Part model, mm, in its own coordinate system. A direction names the side the tool comes from. Coordinates: 2 decimals unless noted, no trailing zeros. Loops run counter-clockwise (first coordinate to the right, second up) from the corner with the lowest first, then second, coordinate; pieces in that order, holes last. Notation, with made-up numbers: M -34,-18.75 L 1,-18.75 A29 cw 1,4.25 Z; hole C 84.25,61 d5. An arc over 180 degrees is marked long. Use CSV: the item, a comma, the result in double quotes. Start each with the question number.
from build123d import *

# Parameters (mm, degrees)
SKETCH1_W                      = 60
SKETCH1_H                      = 42
BOSS_EXTRUDE1_DEPTH            = 12
CUT_EXTRUDE1_REACH             = 14
SKETCH2_R                      = 4
CUT_EXTRUDE1_DIRECTION_2_DEPTH = 1
SKETCH3_R                      = 8
SKETCH3_R_2                    = 4
CUT_EXTRUDE2_DEPTH             = 1
CUT_EXTRUDE2_DEPTH_BACK        = 10
CHAMFER1_SIZE                  = 13
CUT_EXTRUDE4_REACH             = 14
SKETCH5_W                      = 7
SKETCH5_H                      = 4
CUT_EXTRUDE4_DIRECTION_2_DEPTH = 1
SKETCH4_R                      = 2.25
CUT_EXTRUDE3_DEPTH             = 7.5


with BuildPart() as part:
    # Sketch1 → Boss-Extrude1 (new body)
    with BuildSketch(Plane(origin=(0, 0, 0), x_dir=(1, 0, 0), z_dir=(0, 1, 0))):
        Rectangle(SKETCH1_W, SKETCH1_H)
    extrude(amount=BOSS_EXTRUDE1_DEPTH)

    # Sketch2 → Cut-Extrude1 (cut, up to next)
    with BuildSketch(Plane(origin=(0, 12, 0), x_dir=(1, 0, 0), z_dir=(0, 1, 0)), mode=Mode.PRIVATE) as cut_extrude1_sk1:
        Circle(SKETCH2_R)
    cut_extrude1_tool1 = extrude(cut_extrude1_sk1.sketch, amount=-CUT_EXTRUDE1_REACH, mode=Mode.PRIVATE) & part.part
    add(cut_extrude1_tool1.solids().sort_by_distance((0, 12, 0))[0], mode=Mode.SUBTRACT)

    # Sketch2 → Cut-Extrude1 direction 2 (cut)
    with BuildSketch(Plane(origin=(0, 12, 0), x_dir=(1, 0, 0), z_dir=(0, 1, 0))):
        Circle(SKETCH2_R)
    extrude(amount=CUT_EXTRUDE1_DIRECTION_2_DEPTH, mode=Mode.SUBTRACT)

    # Sketch3 → Cut-Extrude2 (cut, two sides)
    with BuildSketch(Plane(origin=(0, 12, 0), x_dir=(1, 0, 0), z_dir=(0, 1, 0))) as cut_extrude2_sk:
        Circle(SKETCH3_R)
        with Locations((20.75, 0)):
            Circle(SKETCH3_R_2)
        with Locations((-20.75, 0)):
            Circle(SKETCH3_R_2)
    extrude(amount=CUT_EXTRUDE2_DEPTH, mode=Mode.SUBTRACT)
    extrude(cut_extrude2_sk.sketch, amount=-CUT_EXTRUDE2_DEPTH_BACK, mode=Mode.SUBTRACT)

    # Chamfer1
    chamfer1_edges = [part.edges().sort_by_distance(p)[0] for p in [
        (30, 6, 21),
        (-30, 6, 21),
    ]]
    chamfer(chamfer1_edges, length=CHAMFER1_SIZE)

    # Sketch5 → Cut-Extrude4 (cut, up to next)
    with BuildSketch(Plane(origin=(0, 12, 0), x_dir=(1, 0, 0), z_dir=(0, 1, 0)), mode=Mode.PRIVATE) as cut_extrude4_sk1:
        with Locations((24, 15)):
            Rectangle(SKETCH5_W, SKETCH5_H)
    cut_extrude4_tool1 = extrude(cut_extrude4_sk1.sketch, amount=-CUT_EXTRUDE4_REACH, mode=Mode.PRIVATE) & part.part
    add(cut_extrude4_tool1.solids().sort_by_distance((24, 12, -15))[0], mode=Mode.SUBTRACT)
    # Sketch5 → Cut-Extrude4 (cut, up to next)
    with BuildSketch(Plane(origin=(0, 12, 0), x_dir=(1, 0, 0), z_dir=(0, 1, 0)), mode=Mode.PRIVATE) as cut_extrude4_sk2:
        with Locations((6, 15)):
            Rectangle(SKETCH5_W, SKETCH5_H)
    cut_extrude4_tool2 = extrude(cut_extrude4_sk2.sketch, amount=-CUT_EXTRUDE4_REACH, mode=Mode.PRIVATE) & part.part
    add(cut_extrude4_tool2.solids().sort_by_distance((6, 12, -15))[0], mode=Mode.SUBTRACT)
    # Sketch5 → Cut-Extrude4 (cut, up to next)
    with BuildSketch(Plane(origin=(0, 12, 0), x_dir=(1, 0, 0), z_dir=(0, 1, 0)), mode=Mode.PRIVATE) as cut_extrude4_sk3:
        with Locations((-6, 15)):
            Rectangle(SKETCH5_W, SKETCH5_H)
    cut_extrude4_tool3 = extrude(cut_extrude4_sk3.sketch, amount=-CUT_EXTRUDE4_REACH, mode=Mode.PRIVATE) & part.part
    add(cut_extrude4_tool3.solids().sort_by_distance((-6, 12, -15))[0], mode=Mode.SUBTRACT)
    # Sketch5 → Cut-Extrude4 (cut, up to next)
    with BuildSketch(Plane(origin=(0, 12, 0), x_dir=(1, 0, 0), z_dir=(0, 1, 0)), mode=Mode.PRIVATE) as cut_extrude4_sk4:
        with Locations((-24, 15)):
            Rectangle(SKETCH5_W, SKETCH5_H)
    cut_extrude4_tool4 = extrude(cut_extrude4_sk4.sketch, amount=-CUT_EXTRUDE4_REACH, mode=Mode.PRIVATE) & part.part
    add(cut_extrude4_tool4.solids().sort_by_distance((-24, 12, -15))[0], mode=Mode.SUBTRACT)

    # Sketch5 → Cut-Extrude4 direction 2 (cut)
    with BuildSketch(Plane(origin=(0, 12, 0), x_dir=(1, 0, 0), z_dir=(0, 1, 0))):
        with Locations((24, 15)):
            Rectangle(SKETCH5_W, SKETCH5_H)
        with Locations((6, 15)):
            Rectangle(SKETCH5_W, SKETCH5_H)
        with Locations((-6, 15)):
            Rectangle(SKETCH5_W, SKETCH5_H)
        with Locations((-24, 15)):
            Rectangle(SKETCH5_W, SKETCH5_H)
    extrude(amount=CUT_EXTRUDE4_DIRECTION_2_DEPTH, mode=Mode.SUBTRACT)

    # Sketch4 → Cut-Extrude3 (cut)
    with BuildSketch(Plane(origin=(0, 0, -21), x_dir=(-1, 0, 0), z_dir=(0, 0, -1))):
        with Locations((-24, 6)):
            Circle(SKETCH4_R)
        with Locations((-6, 6)):
            Circle(SKETCH4_R)
        with Locations((6, 6)):
            Circle(SKETCH4_R)
        with Locations((24, 6)):
            Circle(SKETCH4_R)
    extrude(amount=-CUT_EXTRUDE3_DEPTH, mode=Mode.SUBTRACT)


solid = part.part
1. Wall check: probe 1 along X at (y, z) = (8.75, 0); probe 2 along Z at (x, y) = (8.5, 10.25); probe 3 along Y at (x, z) = (24, -18). Give the ranges that are in metal, low to high.
2. Two-plate mould, pull along Y, no slides. Class faces 1 (the face through (0, 6, 21)), 2 (the face through (-26.146, 6.676, -19.028)), 3 (the face through (-4, 2, 2)): pulls with the +Y half, pulls with the -Y half, needs draft (parallel to the pull), parting line crosses it, or undercut.
3. Tool access for faces 4 (the face through (0, 0, -5)), 5 (the face through (6, 6, -13)), 6 (the face through (-7, 12, -5)), 7 (the face through (-8.146, 6.676, -19.028)), 8 (the face through (-21, 2, 0)): list every direction of +Z, -Z, +X, -X, +Y, -Y with a clear straight run to the whole face (end or side of a thin tool).
4. Slice it at A-A, the plane x = 0. List the corners of the cut face in (y, z), and give its area (3 significant figures).
5. Pin check, flat tips, straight feed: pin 1 (7 mm diameter, centred on x = -24, y = 6, fed in from +Z); pin 2 (8 mm diameter, centred on x = 2, z = -2, fed in from +Y); pin 3 (3.5 mm diameter, centred on x = -24, y = 7.5, fed in from +Z). Stop position of each tip, or through.
6. Slice it at C-C, the plane z = 0. List the corners of the cut face in (x, y).
7. Slice it at B-B, the plane z = -15.5. List the corners of the cut face in (x, y), and give its area (3 significant figures).
8. Slice it at D-D, the plane y = 10.5. List the corners of the cut face in (x, z), and give its area (3 significant figures).
Found:
1,probe 1,"-30 to -24.75, -16.75 to -8, 8 to 16.75, 24.75 to 30"
1,probe 2,"-21 to -17, -13 to 21"
1,probe 3,"0 to 3.75, 8.25 to 12"
2,face 1,"needs draft"
2,face 2,"undercut"
2,face 3,"pulls with the +Y half"
3,face 4,"+Z, -Z, +X, -X, -Y"
3,face 5,"+Y, -Y"
3,face 6,"+Z, -Z, +X, -X, +Y"
3,face 7,"-Z"
3,face 8,"+Y"
4,outline,"M 0,-21 L 12,-21 L 12,-8 L 2,-8 L 2,-4 L 0,-4 Z; M 0,4 L 2,4 L 2,8 L 12,8 L 12,21 L 0,21 Z"
4,area,"328 mm^2"
5,pin 1,"z = 17.5"
5,pin 2,"y = 2"
5,pin 3,"z = 15.75"
6,outline,"M -30,0 L -4,0 L -4,2 L -8,2 L -8,12 L -16.75,12 L -16.75,2 L -24.75,2 L -24.75,12 L -30,12 Z; M 4,0 L 30,0 L 30,12 L 24.75,12 L 24.75,2 L 16.75,2 L 16.75,12 L 8,12 L 8,2 L 4,2 Z"
7,outline,"M -30,0 L -27.5,0 L -27.5,12 L -30,12 Z; M -20.5,0 L -9.5,0 L -9.5,12 L -20.5,12 Z; M -2.5,0 L 2.5,0 L 2.5,12 L -2.5,12 Z; M 9.5,0 L 20.5,0 L 20.5,12 L 9.5,12 Z; M 27.5,0 L 30,0 L 30,12 L 27.5,12 Z"
7,area,"384 mm^2"
8,outline,"M -30,-21 L 30,-21 L 30,8 L 17,21 L -17,21 L -30,8 Z; hole M -27.5,-17 L -20.5,-17 L -20.5,-13 L -27.5,-13 Z; hole C -20.75,0 d8; hole M -9.5,-17 L -2.5,-17 L -2.5,-13 L -9.5,-13 Z; hole C 0,0 d16; hole M 2.5,-17 L 9.5,-17 L 9.5,-13 L 2.5,-13 Z; hole C 20.75,0 d8; hole M 20.5,-17 L 27.5,-17 L 27.5,-13 L 20.5,-13 Z"
8,area,"1,940 mm^2"
